from build123d import *

# Parameters (mm, degrees)
SKETCH1_R            = 3.3782
BOSS_EXTRUDE1_DEPTH  = 3.175
BOSS_EXTRUDE2_DEPTH  = 4.445
SKETCH7_W            = 18.542
SKETCH7_H            = 15.24
BOSS_EXTRUDE4_DEPTH  = 8.43915
SKETCH8_R            = 1.4605
CUT_EXTRUDE3_DEPTH   = 37.635615509
SKETCH9_R            = 10.16
CUT_EXTRUDE4_DEPTH   = 37.635615509
CUT_EXTRUDE6_DEPTH   = 9.525
SKETCH23_R           = 4.490128061
CUT_EXTRUDE7_DEPTH   = 6.35
BOSS_EXTRUDE10_DEPTH = 3.175
BOSS_EXTRUDE11_DEPTH = 3.175
SKETCH19_W           = 8.382
SKETCH19_H           = 4.445
BOSS_EXTRUDE12_DEPTH = 20.32
BOSS_EXTRUDE13_DEPTH = 4.445
CUT_EXTRUDE5_DEPTH   = 12.7
SKETCH24_W           = 48.736365122
SKETCH24_H           = 10.862134757
CUT_EXTRUDE8_DEPTH   = 30.48
SKETCH26_W           = 11.43
SKETCH26_H           = 10.16
BOSS_EXTRUDE15_DEPTH = 3.175
CHAMFER1_SIZE        = 4.445
FILLET1_R            = 3.175


with BuildPart() as part:
    # Sketch1 → Boss-Extrude1 (new body)
    with BuildSketch(Plane(origin=(0, 0, 0), x_dir=(1, 0, 0), z_dir=(0, 1, 0))):
        with BuildLine():
            Line((0, -13.335), (25.4, -13.335))
            Line((25.4, -13.335), (25.4, 13.335))
            Line((25.4, 13.335), (0, 13.335))
            ThreePointArc((0, 13.335), (-13.335, 0), (0, -13.335))
        make_face()
        with Locations(Location((0, 0, 0), (0, 0, 270))):
            Circle(SKETCH1_R, mode=Mode.SUBTRACT)
    boss_extrude1 = extrude(amount=BOSS_EXTRUDE1_DEPTH)

    # Sketch2 → Boss-Extrude2 (add)
    with BuildSketch(Plane(origin=(0, 0, 0), x_dir=(-1, 0, 0), z_dir=(0, -1, 0))):
        Polygon((-25.4, 13.335), (-25.4, -13.335), (-13.335, -13.335), (-13.335, 0), (-13.335, 13.335), align=None)
    extrude(amount=BOSS_EXTRUDE2_DEPTH)

    # Mirror2: Boss-Extrude1 across plane
    add(boss_extrude1.mirror(Plane(origin=(0, -2.2225, 0), x_dir=(0, 0, 1), z_dir=(0, -1, 0))))

    # Sketch7 → Boss-Extrude4 (add)
    with BuildSketch(Plane(origin=(0, -7.62, 0), x_dir=(-1, 0, 0), z_dir=(0, -1, 0))):
        with Locations((-16.129, 0)):
            Rectangle(SKETCH7_W, SKETCH7_H)
    extrude(amount=BOSS_EXTRUDE4_DEPTH)

    # Sketch8 → Cut-Extrude3 (cut, through all)
    with BuildSketch(Plane(origin=(0, 0, -7.62), x_dir=(-1, 0, 0), z_dir=(0, 0, -1))):
        with Locations((-20.7645, -12.1285)):
            Circle(SKETCH8_R)
        with Locations((-11.4935, -12.1285)):
            Circle(SKETCH8_R)
    extrude(amount=-CUT_EXTRUDE3_DEPTH, mode=Mode.SUBTRACT)

    # Sketch9 → Cut-Extrude4 (cut, through all)
    with BuildSketch(Plane(origin=(0, 0, -7.62), x_dir=(-1, 0, 0), z_dir=(0, 0, -1))):
        with Locations((-16.129, -23.67915)):
            Circle(SKETCH9_R)
    extrude(amount=-CUT_EXTRUDE4_DEPTH, mode=Mode.SUBTRACT)

    # Sketch22 → Cut-Extrude6 (cut)
    with BuildSketch(Plane(origin=(0, 3.175, 0), x_dir=(1, 0, 0), z_dir=(0, 1, 0))):
        Polygon((19.3675, -4.490128061), (23.857563833, 0.024016226), (19.3675, 4.490128061), (14.877436167, -0.024016226), align=None)
    extrude(amount=-CUT_EXTRUDE6_DEPTH, mode=Mode.SUBTRACT)

    # Sketch23 → Cut-Extrude7 (cut)
    with BuildSketch(Plane(origin=(0, -6.35, 0), x_dir=(1, 0, 0), z_dir=(0, 1, 0))):
        with Locations(Location((19.3675, 0, 0), (0, 0, 270))):
            Circle(SKETCH23_R)
    extrude(amount=CUT_EXTRUDE7_DEPTH, mode=Mode.SUBTRACT)

    # Sketch16 → Boss-Extrude10 (add)
    with BuildSketch(Plane(origin=(0, 3.175, 0), x_dir=(1, 0, 0), z_dir=(0, 1, 0))):
        Polygon((0, 13.335), (-13.335, 0), (-13.335, 13.335), align=None)
    boss_extrude10 = extrude(amount=-BOSS_EXTRUDE10_DEPTH)

    # Sketch17 → Boss-Extrude11 (add)
    with BuildSketch(Plane.XZ.offset(7.62)):
        Polygon((-13.335, -13.335), (-13.335, 0), (0, -13.335), align=None)
    boss_extrude11 = extrude(amount=-BOSS_EXTRUDE11_DEPTH)

    # Sketch19 → Boss-Extrude12 (add)
    with BuildSketch(Plane(origin=(0, 3.175, 0), x_dir=(1, 0, 0), z_dir=(0, 1, 0))):
        with Locations((-2.5019, 11.1125)):
            Rectangle(SKETCH19_W, SKETCH19_H)
    boss_extrude12 = extrude(amount=BOSS_EXTRUDE12_DEPTH)

    # Sketch20 → Boss-Extrude13 (add)
    with BuildSketch(Plane.XY.offset(-8.89)):
        Polygon((-6.6929, 23.495), (-13.335, 3.175), (-6.6929, 3.175), align=None)
    boss_extrude13 = extrude(amount=-BOSS_EXTRUDE13_DEPTH)

    # Sketch21 → Cut-Extrude5 (cut)
    with BuildSketch(Plane.XY.offset(-8.89)):
        Polygon((0, 22.225), (1.6891, 21.610217877), (1.6891, 20.299782123), (0, 19.685), align=None)
    cut_extrude5 = extrude(amount=-CUT_EXTRUDE5_DEPTH, mode=Mode.SUBTRACT)

    # Mirror3: Boss-Extrude10, Boss-Extrude11, Boss-Extrude12, Boss-Extrude13, Cut-Extrude5 across plane
    add(boss_extrude10.mirror(Plane.XY))
    add(boss_extrude11.mirror(Plane.XY))
    add(boss_extrude12.mirror(Plane.XY))
    add(boss_extrude13.mirror(Plane.XY))
    add(cut_extrude5.mirror(Plane.XY), mode=Mode.SUBTRACT)

    # Sketch24 → Cut-Extrude8 (cut)
    with BuildSketch(Plane(origin=(0, 3.175, 0), x_dir=(1, 0, 0), z_dir=(0, 1, 0))):
        with Locations((2.598122841, 11.203809408)):
            Rectangle(SKETCH24_W, SKETCH24_H)
    extrude(amount=CUT_EXTRUDE8_DEPTH, mode=Mode.SUBTRACT)

    # Sketch26 → Boss-Extrude15 (add)
    with BuildSketch(Plane(origin=(0, 3.175, 0), x_dir=(1, 0, 0), z_dir=(0, 1, 0))):
        with Locations((0, 18.415)):
            Rectangle(SKETCH26_W, SKETCH26_H)
        Polygon((4.490128061, 18.415), (0.007864628, 13.924878827), (-4.490128061, 18.415), (-0.007864628, 22.905121173), align=None, mode=Mode.SUBTRACT)
    extrude(amount=-BOSS_EXTRUDE15_DEPTH)

    # Chamfer1
    chamfer1_edges = [part.edges().sort_by_distance(p)[0] for p in [
        (5.715, 1.5875, -23.495),
        (-5.715, 1.5875, -23.495),
    ]]
    chamfer(chamfer1_edges, length=CHAMFER1_SIZE)

    # Fillet1
    # the kernel refuses this fillet: 3.175 mm, written as the material it adds along each edge
    with BuildSketch(Plane(origin=(-5.715, 3.175, -13.335), x_dir=(0, 0, -1), z_dir=(0, -1, 0))) as fillet1_piece_1:
        with BuildLine():
            CenterArc((FILLET1_R, -FILLET1_R), FILLET1_R, 90, 90)
            Line((0, -FILLET1_R), (0, 0))
            Line((0, 0), (FILLET1_R, 0))
        make_face()
    extrude(amount=3.175)
    with BuildSketch(Plane(origin=(5.715, 3.175, -13.335), x_dir=(0, 0, -1), z_dir=(0, -1, 0))) as fillet1_piece_2:
        with BuildLine():
            CenterArc((FILLET1_R, FILLET1_R), FILLET1_R, 180, 90)
            Line((0, FILLET1_R), (0, 0))
            Line((0, 0), (FILLET1_R, 0))
        make_face()
    extrude(amount=3.175)
    # the kernel refuses this fillet: 3.175 mm, written as the material it takes off along each edge
    with BuildSketch(Plane(origin=(-13.335, 11.1125, -13.335), x_dir=(1, 0, 0), z_dir=(0, -1, 0))) as fillet1_2_piece_1:
        with BuildLine():
            CenterArc((FILLET1_R, FILLET1_R), FILLET1_R, 180, 90)
            Line((0, FILLET1_R), (0, 0))
            Line((0, 0), (FILLET1_R, 0))
        make_face()
    extrude(amount=19.05, mode=Mode.SUBTRACT)
    with BuildSketch(Plane(origin=(-13.335, -15.5575, -13.335), x_dir=(1, 0, 0), z_dir=(0, 1, 0))) as fillet1_2_piece_2:
        with BuildLine():
            CenterArc((FILLET1_R, -FILLET1_R), FILLET1_R, 90, 90)
            Line((0, -FILLET1_R), (0, 0))
            Line((0, 0), (FILLET1_R, 0))
        make_face()
    extrude(amount=19.05, mode=Mode.SUBTRACT)
    with BuildSketch(Plane(origin=(-1.27, 6.462820151, -23.495), x_dir=(1, 0, 0), z_dir=(0, -1, 0)), Plane(origin=(-5.715, 6.462820151, -19.05), x_dir=(0.7071067811865476, 0, -0.7071067811865476), z_dir=(0, -1, 0)), Plane(origin=(1.27, 6.462820151, -23.495), x_dir=(0.7071067811865479, 0, 0.7071067811865472), z_dir=(0, -1, 0)), Plane(origin=(5.715, 6.462820151, -19.05), x_dir=(0, 0, 1), z_dir=(0, -1, 0))) as fillet1_2_piece_3:
        with BuildLine():
            CenterArc((FILLET1_R * 0.414213562373, FILLET1_R), FILLET1_R, 225, 45)
            Line((-FILLET1_R * 0.292893218813, FILLET1_R * 0.292893218813), (0, 0))
            Line((0, 0), (FILLET1_R * 0.414213562373, 0))
        make_face()
    extrude(amount=9.750640303, mode=Mode.SUBTRACT)


solid = part.part
Geometry check sheet. Reference: the model listing, model coordinates, mm. A direction names the side the tool comes from. Give positions to 0.01 mm unless a question says otherwise; leave off trailing zeros. Loops run counter-clockwise (first coordinate to the right, second up) from the corner with the lowest first, then second, coordinate; pieces in that order, holes last. Notation, with made-up numbers: M 38.25,-29 L 80.25,-29 A23 ccw 80.25,4 Z; hole C 59,-22.5 d11. An arc over 180 degrees is marked long. Answer as a JSON object with one key per item and string values. Group by question number.
Item 1: Sectioned sample at D-D on y = 5. Record the boundary of the cut face in (x, z) (3 decimals).
Item 2: Mould release check, pull along X, two halves, no side actions. Record for faces 1 (the flat face through (2, -7.62, -3)), 2 (the cylindrical face through (-5.48, 1.61, -18.93)), 3 (the flat face through (17, 0, 3)): pulls with the +X half, pulls with the -X half, needs draft (parallel to the pull), parting line crosses it, or undercut.
Item 3: Sectioned sample at A-A on z = 2.5. Give the number of separate pieces and of enclosed holes in the cut face, plus the area to 3 significant figures.
Item 4: Access from +Z, -Z, +X, -X, +Y, -Y to the whole of each face (thin tool, end or side, straight path). Record for faces 4 (the flat face through (17.15, 1.61, -2.26)), 5 (the flat face through (22, 0, -3)), 6 (the flat face through (16, -11, 7.62)), 7 (the flat face through (1.689, 12, 11)), 8 (the flat face through (5.715, 2, -17)).
Item 5: Sectioned sample at B-B on x = -1. Record the boundary of the cut face in (y, z) (3 decimals), plus the area to 3 significant figures.
Item 6: Gauge pin test, flat ends, axial feed: pin 1 (1 mm diameter, centred on x = -9.5, y = 1, fed in from -Z) (3 decimals); pin 2 (9.5 mm diameter, centred on x = 14, y = -13, fed in from -Z); pin 3 (0.6 mm diameter, centred on y = 2, z = -17, fed in from -X) (3 decimals). Record the tip position at first contact, or that the pin passes through.
Item 7: Material ranges on L1, parallel to X at y = -5, z = 0 (3 decimals); L2, parallel to Y at x = -7, z = -13 (3 decimals); L3, parallel to X at y = 1, z = -0.5 (3 decimals), recorded low to high.
Item 8: Sectioned sample at C-C on y = -9. Record the boundary of the cut face in (x, z).
Findings below:
{
 "1": {"outline": "M -12.738,8.89 L 1.689,8.89 L 1.689,13.335 L -12.738,13.335 Z"},
 "2": {"face 1": "needs draft", "face 2": "pulls with the -X half", "face 3": "undercut"},
 "3": {"separate pieces": "3", "enclosed holes": "2", "area": "330 mm2"},
 "4": {"face 4": "+Y", "face 5": "none", "face 6": "+Z, +X, -X, -Y", "face 7": "+Z, -Z, +X, +Y", "face 8": "-Z, +X, +Y, -Y"},
 "5": {"outline": "M -7.62,-13.335 L -4.445,-13.335 L -4.445,-3.227 L -7.62,-3.227 Z; M -7.62,3.227 L -4.445,3.227 L -4.445,13.335 L -7.62,13.335 Z; M 0,-23.318 L 3.175,-23.318 L 3.175,-21.911 L 0,-21.911 Z; M 0,-14.931 L 3.175,-14.931 L 3.175,-3.227 L 0,-3.227 Z; M 0,3.227 L 3.175,3.227 L 3.175,8.89 L 23.495,8.89 L 23.495,13.335 L 0,13.335 Z", "area": "228 mm2"},
 "6": {"pin 1": "z = -13.335", "pin 2": "z = -7.62", "pin 3": "x = -5.715"},
 "7": {"L1": "-13.335 to -3.378, 3.378 to 14.877, 23.858 to 25.4", "L2": "-7.62 to -4.445, 0 to 3.175", "L3": "-13.335 to -3.341, 3.341 to 15.399, 23.379 to 25.4"},
 "8": {"outline": "M 6.86,-7.62 L 25.4,-7.62 L 25.4,7.62 L 6.86,7.62 Z"}
}
